Geometry: final body of the model. Coordinates: model frame, mm. Face numbers are marked on the shaded views. Coordinates: 2 decimals unless noted, no trailing zeros. Write each loop counter-clockwise with the first axis right and the second up, starting at its lowest first coordinate (ties: lowest second). Pieces come first, ordered by that corner, then holes. Notation, with made-up numbers: (-14.5, 68) - (41.5, 68) arc R18 cw to (41.5, 91) - close; hole circle Ø9 at (73.5, 42.5). An arc over 180 degrees is marked (long way). Answer as a JSON object with one key per item and string values. Group by question number.
Item 1: Section A-A on z = 10.5. Return loops of the section in (x, y), and give its area (3 significant figures).
Item 2: Mould query, pull axis X, two halves, no side actions, for the marked faces 1, 2 and 3. Classes: pulls with the +X half, pulls with the -X half, needs draft (parallel to the pull), parting line crosses it, or undercut.
Item 3: Line query: line 1 along Z through (x, y) = (-15.5, -31.5); line 2 along Y through (x, z) = (-10, 16); line 3 along X through (y, z) = (-35.5, 14.5). Output: solid intervals per line, ascending. Write a range as from..to.
Item 4: First-contact query: pin 1 Ø1.5 at (x, z) = (4, 12.5) entering from +Y; pin 2 Ø5.5 at (x, z) = (46.5, 21.5) entering from +Y; pin 3 Ø2.5 at (x, z) = (-48, 21.5) entering from -Y; pin 4 Ø5.5 at (x, y) = (-25.5, -40.5) entering from -Z. Flat tips, straight axial feed; report the tip coordinate or a pass-through.
```python
from build123d import *

# Parameters (mm, degrees)
F0_R     = 12
F1_DEPTH = 3
F2_DEPTH = 23
F4_START = 18
F4_DEPTH = 5
F5_SIZE  = 3


with BuildPart() as f1:
    # F0 (on Top) → F1 (new body)
    with BuildSketch(Plane.XY):
        with BuildLine():
            ThreePointArc((0, -50), (35.3553390593, -35.3553390593), (50, 0))
            ThreePointArc((50, 0), (-35.3553390593, 35.3553390593), (0, -50))
        make_face()
        Circle(F0_R, mode=Mode.SUBTRACT)
    extrude(amount=F1_DEPTH)

    # F0 (on Top) → F2 (join)
    with BuildSketch(Plane.XY):
        with BuildLine():
            ThreePointArc((52.5, 0), (-37.1231060123, 37.1231060123), (0, -52.5))
            ThreePointArc((0, -52.5), (37.1231060123, -37.1231060123), (52.5, 0))
        make_face()
        with BuildLine():
            ThreePointArc((0, -50), (-35.3553390593, 35.3553390593), (50, 0))
            ThreePointArc((50, 0), (35.3553390593, -35.3553390593), (0, -50))
        make_face(mode=Mode.SUBTRACT)
    extrude(amount=F2_DEPTH)

    # F3 (on Top) → F4 (join)
    with BuildSketch(Plane.XY.offset(F4_START)):
        with BuildLine():
            Line((31.8198051534, -31.8198051534), (35.3553390593, -35.3553390593))
            ThreePointArc((35.3553390593, -35.3553390593), (46.1939766256, -19.1341716183), (50, 0))
            Line((50, 0), (45, 0))
            ThreePointArc((45, 0), (41.574578963, -17.2207544564), (31.8198051534, -31.8198051534))
        make_face()
        with BuildLine():
            ThreePointArc((-45, 0), (-41.574578963, 17.2207544564), (-31.8198051534, 31.8198051534))
            Line((-31.8198051534, 31.8198051534), (-35.3553390593, 35.3553390593))
            ThreePointArc((-35.3553390593, 35.3553390593), (-46.1939766256, 19.1341716183), (-50, 0))
            Line((-50, 0), (-45, 0))
        make_face()
        with BuildLine():
            ThreePointArc((35.3553390593, 35.3553390593), (19.1341716183, 46.1939766256), (0, 50))
            Line((0, 50), (0, 45))
            ThreePointArc((0, 45), (17.2207544564, 41.574578963), (31.8198051534, 31.8198051534))
            Line((31.8198051534, 31.8198051534), (35.3553390593, 35.3553390593))
        make_face()
        with BuildLine():
            Line((-31.8198051534, -31.8198051534), (-35.3553390593, -35.3553390593))
            ThreePointArc((-35.3553390593, -35.3553390593), (-19.1341716183, -46.1939766256), (0, -50))
            Line((0, -50), (0, -45))
            ThreePointArc((0, -45), (-17.2207544564, -41.574578963), (-31.8198051534, -31.8198051534))
        make_face()
    extrude(amount=F4_DEPTH)

    # F5
    f5_edges = [f1.edges().sort_by_distance(p)[0] for p in [
        (0, 52.5, 0),
    ]]
    chamfer(f5_edges, length=F5_SIZE)


solid = f1.part
```
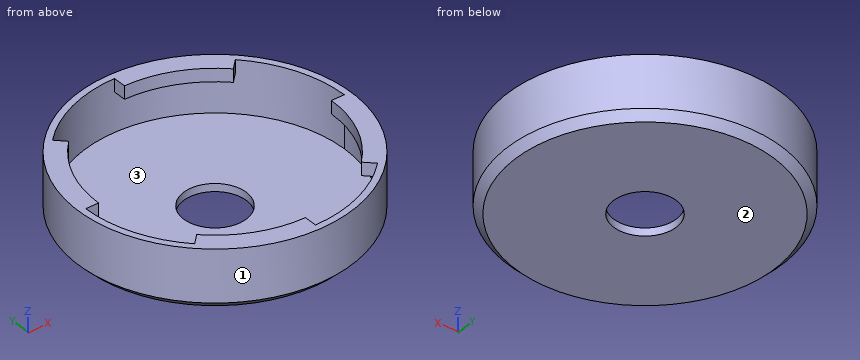
Checks:
{
 "1": {"outline": "circle Ø105 at (0, 0); hole circle Ø100 at (0, 0)", "area": "805 mm^2"},
 "2": {"face 1": "parting line crosses it", "face 2": "needs draft", "face 3": "undercut"},
 "3": {"line 1": "0..3", "line 2": "-51.54..-48.99, 48.99..51.54", "line 3": "-38.68..-35.21, 35.21..38.68"},
 "4": {"pin 1": "y = 52.4", "pin 2": "y = 29.02", "pin 3": "y = -23.89", "pin 4": "z = 0"}
}
